Work out the finished part from the listing and answer in its coordinate system (mm). A direction names the side the tool comes from. Round coordinates to 2 decimals unless told otherwise and drop trailing zeros. Order: outer loops, then holes, each group sorted by start corner. A loop starts at its lowest first (then second) coordinate and runs counter-clockwise, first axis right, second up. Notation, with made-up numbers: (-28, 16.25) -> (25, 16.25) arc R27 cw to (25, 42.25) -> close; hole circle Ø4 at (80, 68). An arc over 180 degrees is marked (long way). Use a Markdown table: item, result. Add a question column.
Item 1: For a pull along Z with two mould halves and no side action, classify faces 1 (the flat face through (11, 35, 30)), 2 (the cylindrical face through (7.352, -4.213, 4.839)), 3 (the flat face through (27.25, 72, 15)) as +Z half, -Z half, draft (parallel to the pull), parting line (faces both ways), or undercut.
Item 2: Find the intervals of material crossed by L1, parallel to Z at x = 32, y = 90; L2, parallel to Y at x = 9.25, z = 15; L3, parallel to X at y = 79, z = 4, in increasing order. Write a range as [from, to].
Item 3: A cutting plane is placed at A-A, the plane z = 15. Give the number of separate pieces and of enclosed holes in the cut face, plus the area to 4 significant figures.
Item 4: A cutting plane is placed at B-B, the plane y = 42.5. Determine the outline of the cut face in (x, z), plus the area to 3 significant figures.
Item 5: A cutting plane is placed at C-C, the plane x = 4. Determine the outline of the cut face in (y, z).
Item 6: Flat-ended cylindrical pins translate along their axes: P1, Ø4.5, axis at x = 10, z = 7.5, coming from the +Y side; P2, Ø15, axis at y = 91, z = 16.5, coming from the +X side; P3, Ø10, axis at x = -4, z = 16.5, coming from the -Y side; P4, Ø1, axis at x = 3.5, z = 20.5, coming from the -Y side. Find the tip coordinate at first contact, or state that the pin passes through.
Item 7: A tool of negligible diameter and unlimited length cuts with its end or side. For faces 4 (the cylindrical face through (32.21, 97.54, 20.78)), 5 (the flat face through (-6.46, 43.71, 15.21)), 6 (the cylindrical face through (-17.79, 97.54, 9.22)), from which of +Z, -Z, +X, -X, +Y, -Y can it reach the whole face along a straight path? Write none if from no direction.
Item 8: A cutting plane is placed at D-D, the plane y = 92. Determine the outline of the cut face in (x, z).
from build123d import *

# Parameters (mm, degrees)
EXTRUDE_1_DEPTH     = 30
CUT_EXTRUDE_1_DEPTH = 102.205545797
EXTRUDE_2_DEPTH     = 14.5
SKETCH_4_R          = 11
CUT_EXTRUDE_2_DEPTH = 20
EXTRUDE_3_DEPTH     = 8
EXTRUDE_START       = -8
EXTRUDE_4_DEPTH     = 8
SKETCH_9_R          = 7.5
CUT_EXTRUDE_5_DEPTH = 62
SKETCH_10_R         = 9.5
CUT_EXTRUDE_6_DEPTH = 6
CUT_EXTRUDE_START   = -6
SKETCH_11_R         = 9.5
CUT_EXTRUDE_7_DEPTH = 6


with BuildPart() as part:
    # 草图1 → 凸台-拉伸1 (new body)
    with BuildSketch(Plane.XY):
        Polygon((0, 0), (14.5, 0), (14.5, 25), (35.25, 45.75), (35.25, 90), (27.25, 90), (27.25, 50), (-12.75, 50), (-12.75, 90), (-20.75, 90), (-20.75, 45.75), (0, 25), align=None)
    extrude(amount=EXTRUDE_1_DEPTH)

    # 草图2 → 切除-拉伸1 (cut, through all)
    with BuildSketch(Plane.XY.offset(30)):
        Polygon((-12.75, 50), (0, 37.25), (14.5, 37.25), (27.25, 50), align=None)
    extrude(amount=-CUT_EXTRUDE_1_DEPTH, mode=Mode.SUBTRACT)

    # 草图3 → 凸台-拉伸2 (add)
    with BuildSketch(Plane(origin=(14.5, 0, 0), x_dir=(0, 0, -1), z_dir=(1, 0, 0))):
        with BuildLine():
            Line((-30, 0), (0, 0))
            ThreePointArc((0, 0), (-15, -15), (-30, 0))
        make_face()
    extrude(amount=-EXTRUDE_2_DEPTH)

    # 草图4 → 切除-拉伸2 (cut)
    with BuildSketch(Plane(origin=(14.5, 0, 0), x_dir=(0, 0, -1), z_dir=(1, 0, 0))):
        with Locations((-15, 0)):
            Circle(SKETCH_4_R)
    extrude(amount=-CUT_EXTRUDE_2_DEPTH, mode=Mode.SUBTRACT)

    # 草图7 → 凸台-拉伸3 (add)
    with BuildSketch(Plane(origin=(35.25, 0, 0), x_dir=(0, 0, -1), z_dir=(1, 0, 0))):
        with BuildLine():
            Line((-30, 90), (0, 90))
            ThreePointArc((0, 90), (-15, 105), (-30, 90))
        make_face()
    extrude(amount=-EXTRUDE_3_DEPTH)

    # 草图8 → 凸台-拉伸4 (add)
    with BuildSketch(Plane.ZY.offset(20.75).offset(EXTRUDE_START)):
        with BuildLine():
            Line((0, 90), (30, 90))
            ThreePointArc((30, 90), (15, 105), (0, 90))
        make_face()
    extrude(amount=EXTRUDE_4_DEPTH)

    # 草图9 → 切除-拉伸5 (cut)
    with BuildSketch(Plane.ZY.offset(20.75)):
        with Locations(Location((15, 90, 0), (0, 0, 270))):
            Circle(SKETCH_9_R)
    extrude(amount=-CUT_EXTRUDE_5_DEPTH, mode=Mode.SUBTRACT)

    # 草图10 → 切除-拉伸6 (cut)
    with BuildSketch(Plane.ZY.offset(20.75)):
        with Locations(Location((15, 90, 0), (0, 0, 270))):
            Circle(SKETCH_10_R)
    extrude(amount=-CUT_EXTRUDE_6_DEPTH, mode=Mode.SUBTRACT)

    # 草图11 → 切除-拉伸7 (cut)
    with BuildSketch(Plane(origin=(35.25, 0, 0), x_dir=(0, 0, -1), z_dir=(1, 0, 0)).offset(CUT_EXTRUDE_START)):
        with Locations(Location((-15, 90, 0), (0, 0, 270))):
            Circle(SKETCH_11_R)
    extrude(amount=CUT_EXTRUDE_7_DEPTH, mode=Mode.SUBTRACT)


solid = part.part
Reported:
| question | item | result |
|---|---|---|
| 1 | face 1 | +Z half |
| 1 | face 2 | undercut |
| 1 | face 3 | draft |
| 2 | L1 | [0, 5.5], [24.5, 30] |
| 2 | L2 | [-15, -11], [11, 37.25] |
| 2 | L3 | [-20.75, -12.75], [27.25, 35.25] |
| 3 | separate pieces | 4 |
| 3 | enclosed holes | 0 |
| 3 | area | 1,475 mm² |
| 4 | outline | (-17.5, 0) -> (-5.25, 0) -> (-5.25, 30) -> (-17.5, 30) -> close; (19.75, 0) -> (32, 0) -> (32, 30) -> (19.75, 30) -> close |
| 4 | area | 735 mm² |
| 5 | outline | (0, 0) -> (37.25, 0) -> (37.25, 30) -> (0, 30) arc R15 ccw to start; hole circle Ø22 at (0, 15) |
| 6 | P1 | y = 37.25 |
| 6 | P2 | x = 29.25 |
| 6 | P3 | y = -15 |
| 6 | P4 | y = -14.14 |
| 7 | face 4 | +X |
| 7 | face 5 | +Z, -Z, +Y |
| 7 | face 6 | -X |
| 8 | outline | (-20.75, 0.13) -> (-12.75, 0.13) -> (-12.75, 7.77) -> (-14.75, 7.77) -> (-14.75, 5.71) -> (-20.75, 5.71) -> close; (-20.75, 24.29) -> (-14.75, 24.29) -> (-14.75, 22.23) -> (-12.75, 22.23) -> (-12.75, 29.87) -> (-20.75, 29.87) -> close; (27.25, 0.13) -> (35.25, 0.13) -> (35.25, 5.71) -> (29.25, 5.71) -> (29.25, 7.77) -> (27.25, 7.77) -> close; (27.25, 22.23) -> (29.25, 22.23) -> (29.25, 24.29) -> (35.25, 24.29) -> (35.25, 29.87) -> (27.25, 29.87) -> close |
